```python
from build123d import *

# Parameters (mm, degrees)
SKETCH1_R                  = 4
BOSS_EXTRUDE1_DEPTH        = 12.7
CUT_EXTRUDE1_DEPTH         = 94.864476774
CUT_EXTRUDE1_DEPTH_BACK    = 94.864476774
SKETCH2_W                  = 2.7
SKETCH2_H                  = 29.5
M6X1_0_TAPPED_HOLE1_D      = 5
M6X1_0_TAPPED_HOLE1_DEPTH  = 15
M6X1_0_TAPPED_HOLE1_TIP    = 1.502151548
BOSS_EXTRUDE2_DEPTH        = 2
M10X1_5_TAPPED_HOLE1_D     = 8.5
M10X1_5_TAPPED_HOLE1_DEPTH = 10
CUT_EXTRUDE2_DEPTH         = 94.864476774
CUT_EXTRUDE2_DEPTH_BACK    = 94.864476774
SKETCH8_OUTSIDE_W          = 38.158
SKETCH8_OUTSIDE_H          = 101.958
SKETCH8_OUTSIDE_W_2        = 10
SKETCH8_OUTSIDE_H_2        = 76.5


with BuildPart() as part:
    # Sketch1 → Boss-Extrude1 (new body)
    with BuildSketch(Plane.XY):
        with BuildLine():
            Line((-21, 64.5), (-7, 64.5))
            ThreePointArc((-7, 64.5), (-4.071067812, 57.428932188), (3, 54.5))
            Line((3, 54.5), (43, 54.5))
            ThreePointArc((43, 54.5), (50.071067812, 57.428932188), (53, 64.5))
            Line((53, 64.5), (67, 64.5))
            Line((67, 64.5), (67, 49.5))
            ThreePointArc((67, 49.5), (66.299754559, 41.161283045), (64.218631982, 33.056132032))
            Line((64.218631982, 33.056132032), (51.332471676, -3.946528312))
            ThreePointArc((51.332471676, -3.946528312), (46.951318589, -9.781572975), (40, -12))
            Line((40, -12), (0, -12))
            ThreePointArc((0, -12), (-7.623489029, -9.26727657), (-11.77483021, -2.313735836))
            Line((-11.77483021, -2.313735836), (-20.061792543, 39.859434015))
            ThreePointArc((-20.061792543, 39.859434015), (-20.764895394, 44.656944514), (-21, 49.5))
            Line((-21, 49.5), (-21, 64.5))
        make_face()
        Circle(SKETCH1_R, mode=Mode.SUBTRACT)
        with Locations((40, 0)):
            Circle(SKETCH1_R, mode=Mode.SUBTRACT)
        with BuildLine():
            Line((-6.400325135, 32.571886803), (-4.337091454, 22.071886803))
            ThreePointArc((-4.337091454, 22.071886803), (-0.87764047, 16.277269525), (5.475267055, 14))
            Line((5.475267055, 14), (37.768949155, 14))
            ThreePointArc((37.768949155, 14), (43.561714646, 15.848689187), (47.212675552, 20.711226406))
            Line((47.212675552, 20.711226406), (50.869295966, 31.211226406))
            ThreePointArc((50.869295966, 31.211226406), (49.576880383, 40.292765491), (41.42556957, 44.5))
            Line((41.42556957, 44.5), (3.412033373, 44.5))
            ThreePointArc((3.412033373, 44.5), (-4.310697101, 40.852907524), (-6.400325135, 32.571886803))
        make_face(mode=Mode.SUBTRACT)
    extrude(amount=BOSS_EXTRUDE1_DEPTH)

    # Sketch2 → Cut-Extrude1 (cut, two sides: drawn at the far end of the back side and taken through both)
    with BuildSketch(Plane(origin=(0, 0, 0), x_dir=(0, 0, -1), z_dir=(1, 0, 0)).offset(-CUT_EXTRUDE1_DEPTH_BACK)):
        with Locations((-11.35, 2.75)):
            Rectangle(SKETCH2_W, SKETCH2_H)
    extrude(amount=CUT_EXTRUDE1_DEPTH + CUT_EXTRUDE1_DEPTH_BACK, mode=Mode.SUBTRACT)

    # M6x1.0 Tapped Hole1
    with Locations(Plane(origin=(0, 64.5, 0), x_dir=(1, 0, 0), z_dir=(0, 1, 0))):
        with Locations((-14, -3.5), (60, -3.5)):
            Hole(M6X1_0_TAPPED_HOLE1_D / 2, depth=M6X1_0_TAPPED_HOLE1_DEPTH)
            with Locations((0, 0, -(M6X1_0_TAPPED_HOLE1_DEPTH + M6X1_0_TAPPED_HOLE1_TIP / 2))):  # 118° drill point
                Cone(0, M6X1_0_TAPPED_HOLE1_D / 2, M6X1_0_TAPPED_HOLE1_TIP, mode=Mode.SUBTRACT)

    # Sketch5 → Boss-Extrude2 (add)
    with BuildSketch(Plane.XY):
        with BuildLine():
            Line((5.475267055, 14), (37.768949155, 14))
            ThreePointArc((37.768949155, 14), (43.561714646, 15.848689187), (47.212675552, 20.711226406))
            Line((47.212675552, 20.711226406), (50.869295966, 31.211226406))
            ThreePointArc((50.869295966, 31.211226406), (49.576880383, 40.292765491), (41.42556957, 44.5))
            Line((41.42556957, 44.5), (3.412033373, 44.5))
            ThreePointArc((3.412033373, 44.5), (-4.310697101, 40.852907524), (-6.400325135, 32.571886803))
            Line((-6.400325135, 32.571886803), (-4.337091454, 22.071886803))
            ThreePointArc((-4.337091454, 22.071886803), (-0.87764047, 16.277269525), (5.475267055, 14))
        make_face()
    extrude(amount=BOSS_EXTRUDE2_DEPTH)

    # M10x1.5 Tapped Hole1
    with Locations(Plane.XY.offset(10)):
        with Locations((0, 0), (40, 0)):
            Hole(M10X1_5_TAPPED_HOLE1_D / 2, depth=M10X1_5_TAPPED_HOLE1_DEPTH)

    # Sketch8 outside → Cut-Extrude2 (cut, two sides: drawn at the far end of the back side and taken through both)
    with BuildSketch(Plane(origin=(0, 0, 0), x_dir=(0, 0, -1), z_dir=(1, 0, 0)).offset(-CUT_EXTRUDE2_DEPTH_BACK)):
        with Locations((-6.35, 26.25)):
            Rectangle(SKETCH8_OUTSIDE_W, SKETCH8_OUTSIDE_H)
        with Locations((-5, 26.25)):
            Rectangle(SKETCH8_OUTSIDE_W_2, SKETCH8_OUTSIDE_H_2, mode=Mode.SUBTRACT)
    extrude(amount=CUT_EXTRUDE2_DEPTH + CUT_EXTRUDE2_DEPTH_BACK, mode=Mode.SUBTRACT)


solid = part.part
```
Geometry check sheet. Reference: the model listing, model coordinates, mm. A direction names the side the tool comes from. Coordinates: 2 decimals unless noted, no trailing zeros. Order: outer loops, then holes, each group sorted by start corner. A loop starts at its lowest first (then second) coordinate and runs counter-clockwise, first axis right, second up. Notation, with made-up numbers: (-18.5, 52) - (12.5, 52) arc R12 cw to (12.5, 57) - close; hole circle Ø4 at (21.25, -21). An arc over 180 degrees is marked (long way). Answer in a Markdown table with one row per item. Add a question column.
1. Section check B-B (y = 24). Enter the section's corners in (x, z), plus the area to 3 significant figures.
2. Access from +Z, -Z, +X, -X, +Y, -Y to the whole of each face (thin tool, end or side, straight path). Record for faces 1 (the face through (49.653, 40.184, 5.944)), 2 (the face through (-4.15, 57.51, 4.93)), 3 (the face through (44.246, 0.187, 4.93)).
3. Gauge pin test, flat ends, axial feed: pin 1 Ø1 at (x, z) = (14.5, 2) entering from +Y; pin 2 Ø1.5 at (x, y) = (17, 26) entering from +Z; pin 3 Ø7 at (x, y) = (0, 0) entering from -Z; pin 4 Ø6 at (y, z) = (29, 6) entering from -X. Record the tip position at first contact, or that the pin passes through.
4. Section check D-D (y = 12.5). Enter the section's corners in (x, z).
5. Section check C-C (x = 49.5). Enter the section's corners in (y, z), plus the area to 3 significant figures.
6. Section check A-A (z = 7). Enter the section's corners in (x, y).
7. Material ranges on L1, parallel to Z at x = -14, y = 56; L2, parallel to Y at x = 1, z = 4; L3, parallel to Y at x = 16.5, z = 5, recorded low to high. Write a range as [from, to].
8. Draft check along X on faces 4 (the face through (49.015, 25.888, 5.944)), 5 (the face through (-21, 57, 5)), 6 (the face through (22, 27, 0)), 7 (the face through (-0.952, 16.339, 5.944)). Enter one of: +X half, -X half, draft (parallel to the pull), parting line (faces both ways), or undercut.
Data:
| question | item | result |
|---|---|---|
| 1 | outline | (-16.95, 0) - (61.06, 0) - (61.06, 10) - (48.36, 10) - (48.36, 2) - (-4.72, 2) - (-4.72, 10) - (-16.95, 10) - close |
| 1 | area | 356 mm² |
| 2 | face 1 | +Z |
| 2 | face 2 | +Z, -Z, +Y |
| 2 | face 3 | +Z, -Z |
| 3 | pin 1 | stops at y = 54.5 |
| 3 | pin 2 | stops at z = 2 |
| 3 | pin 3 | passes through |
| 3 | pin 4 | stops at x = -18.52 |
| 4 | outline | (-14.69, 0) - (57.06, 0) - (57.06, 10) - (-14.69, 10) - close |
| 5 | outline | (-7.33, 0) - (56.9, 0) - (56.9, 10) - (40.4, 10) - (40.4, 2) - (27.28, 2) - (27.28, 10) - (-7.33, 10) - close |
| 5 | area | 537 mm² |
| 6 | outline | (-21, 49.5) arc R50 ccw to (-20.06, 39.86) - (-11.77, -2.31) arc R12 ccw to (0, -12) - (40, -12) arc R12 ccw to (51.33, -3.95) - (64.22, 33.06) arc R50 ccw to (67, 49.5) - (67, 64.5) - (53, 64.5) arc R10 cw to (43, 54.5) - (3, 54.5) arc R10 cw to (-7, 64.5) - (-21, 64.5) - close; hole (-6.4, 32.57) - (-4.34, 22.07) arc R10 ccw to (5.48, 14) - (37.77, 14) arc R10 ccw to (47.21, 20.71) - (50.87, 31.21) arc R10 ccw to (41.43, 44.5) - (3.41, 44.5) arc R10 ccw to start; hole circle Ø8.5 at (0, 0); hole circle Ø8.5 at (40, 0) |
| 7 | L1 | z = [0, 1], [6, 10] |
| 7 | L2 | y = [-12, -4.13], [4.13, 15.06], [44.2, 54.7] |
| 7 | L3 | y = [-12, 14], [44.5, 54.5] |
| 8 | face 4 | undercut |
| 8 | face 5 | -X half |
| 8 | face 6 | draft |
| 8 | face 7 | undercut |
